```python
from build123d import *

# Parameters (mm, degrees)
F0_R     = 10.875
F0_R_2   = 1.675
F1_DEPTH = 6.7
F2_R     = 4
F3_DEPTH = 2.8
F4_R     = 2.25
F5_DEPTH = 12.5
F6_R     = 0.5


with BuildPart() as f1:
    # F0 (on Top) → F1 (new body)
    with BuildSketch(Plane.XY):
        Circle(F0_R)
        with Locations((-5.853981, -5.072985)):
            Circle(F0_R_2, mode=Mode.SUBTRACT)
        with Locations((5.076866, -5.85559)):
            Circle(F0_R_2, mode=Mode.SUBTRACT)
        with Locations((-5.074026, 5.858051)):
            Circle(F0_R_2, mode=Mode.SUBTRACT)
        with Locations((5.856821, 5.075446)):
            Circle(F0_R_2, mode=Mode.SUBTRACT)
    extrude(amount=F1_DEPTH)

    # F2 (on Top) → F3 (join)
    with BuildSketch(Plane.XY):
        Circle(F2_R)
    extrude(amount=-F3_DEPTH)

    # F4 (on Top) → F5 (cut, symmetric)
    with BuildSketch(Plane.XY):
        Circle(F4_R)
    extrude(amount=F5_DEPTH, both=True, mode=Mode.SUBTRACT)

    # F6
    f6_edges = [f1.edges().sort_by_distance(p)[0] for p in [
        (-4, 0, -2.8),
    ]]
    fillet(f6_edges, radius=F6_R)


solid = f1.part
```
The listing builds one solid part. Answer for the finished solid, in the listing's coordinates (mm). Give positions to 0.01 mm unless a question says otherwise; leave off trailing zeros. Loops run counter-clockwise (first coordinate to the right, second up) from the corner with the lowest first, then second, coordinate; pieces in that order, holes last. Notation, with made-up numbers: M 9.5,40 L 57.5,40 A12 ccw 57.5,54 Z; hole C 26,50 d4. An arc over 180 degrees is marked long. One line per item, written item: value.
1. Find the intervals of material crossed by probe 1 along Y at (x, z) = (0, 2.5) (3 decimals); probe 2 along Y at (x, z) = (5, 5); probe 3 along Y at (x, z) = (-4.5, 5.5), in increasing order.
Found:
probe 1: -10.875 to -2.25, 2.25 to 10.875
probe 2: -9.66 to -7.53, -4.18 to 3.64, 6.51 to 9.66
probe 3: -9.9 to -6.06, -4.09 to 4.28, 7.43 to 9.9
2. Section D-D on x = -5.25 is taken. Determine the outline of the cut face in (y, z), plus the area to 3 significant figures.
Found:
outline: M -9.52,0 L -6.64,0 L -6.64,6.7 L -9.52,6.7 Z; M -3.51,0 L 4.19,0 L 4.19,6.7 L -3.51,6.7 Z; M 7.52,0 L 9.52,0 L 9.52,6.7 L 7.52,6.7 Z
area: 84.4 mm^2
3. For a pull along Y with two mould halves and no side action, classify faces 1 (the face through (5, 0, 0)), 2 (the face through (-0.867, -3.905, -1.134)), 3 (the face through (6.63, 3.59, 3.3)) as pulls with the +Y half, pulls with the -Y half, needs draft (parallel to the pull), parting line crosses it, or undercut.
Found:
face 1: needs draft
face 2: parting line crosses it
face 3: undercut
4. Section A-A on x = 0 is taken. Determine the outline of the cut face in (y, z) (3 decimals), plus the area to 3 significant figures.
Found:
outline: M -10.875,0 L -4,0 L -4,-2.3 A0.5 ccw -3.5,-2.8 L -2.25,-2.8 L -2.25,6.7 L -10.875,6.7 Z; M 2.25,-2.8 L 3.5,-2.8 A0.5 ccw 4,-2.3 L 4,0 L 10.875,0 L 10.875,6.7 L 2.25,6.7 Z
area: 125 mm^2
5. Each of these flat-tipped pins is pushed along its axis until it touches: P1, Ø3, axis at x = 5.86, y = 5.08, coming from the +Z side; P2, Ø4.5, axis at x = -5.07, y = 5.86, coming from the -Z side; P3, Ø3, axis at y = 5.5, z = 5.5, coming from the -X side; P4, Ø5, axis at y = 4, z = -1, coming from the -X side. Where does it stop, or does it pass through?
Found:
P1: through
P2: z = 0
P3: x = -10.11
P4: x = -10.74
6. Section C-C on z = 3.25 is taken. Determine the outline of the cut face in (x, y) (3 decimals).
Found:
outline: C 0,0 d21.75; hole C -5.854,-5.073 d3.35; hole C -5.074,5.858 d3.35; hole C 0,0 d4.5; hole C 5.077,-5.856 d3.35; hole C 5.857,5.075 d3.35
